```python
from build123d import *

# Parameters (mm, degrees)
F0_R     = 5.75
F1_DEPTH = 2.5
F2_R     = 1.375
F3_DEPTH = 25.4
F4_R     = 0.6
F5_DEPTH = 25.4
F6_R     = 0.6
F7_DEPTH = 25.4
F8_R     = 0.6
F9_DEPTH = 25.4
F10_SIZE = 1
F11_R    = 0.4


with BuildPart() as f1:
    # F0 (on Top) → F1 (new body)
    with BuildSketch(Plane.XY):
        with Locations((-19.332174, 0)):
            Circle(F0_R)
    extrude(amount=F1_DEPTH)

    # F2 (on face) → F3 (cut)
    with BuildSketch(Plane.XY.offset(2.5)):
        with Locations((-19.332174, 0)):
            Circle(F2_R)
    extrude(amount=-F3_DEPTH, mode=Mode.SUBTRACT)

    # F4 (on face) → F5 (cut)
    with BuildSketch(Plane.XY.offset(2.5)):
        with Locations((-22.144392, 2.014774)):
            Circle(F4_R)
    extrude(amount=-F5_DEPTH, mode=Mode.SUBTRACT)

    # F6 (on face) → F7 (cut)
    with BuildSketch(Plane.XY.offset(2.5)):
        with Locations((-19.493969, -3.397938)):
            Circle(F6_R)
    extrude(amount=-F7_DEPTH, mode=Mode.SUBTRACT)

    # F8 (on face) → F9 (cut)
    with BuildSketch(Plane.XY.offset(2.5)):
        with Locations((-16.320517, 1.792489)):
            Circle(F8_R)
    extrude(amount=-F9_DEPTH, mode=Mode.SUBTRACT)

    # F10
    f10_edges = [f1.edges().sort_by_distance(p)[0] for p in [
        (-25.082174, 0, 2.5),
    ]]
    chamfer(f10_edges, length=F10_SIZE)

    # F11
    f11_edges = [f1.edges().sort_by_distance(p)[0] for p in [
        (-25.082174, 0, 0),
    ]]
    fillet(f11_edges, radius=F11_R)


solid = f1.part
```
Verification items for the finished model (mm, model axes). Round coordinates to 2 decimals unless told otherwise and drop trailing zeros. Loops run counter-clockwise (first coordinate to the right, second up) from the corner with the lowest first, then second, coordinate; pieces in that order, holes last. Notation, with made-up numbers: (16, -36) -> (24, -36) arc R29 ccw to (24, -14) -> close; hole circle Ø11 at (53.5, 19). An arc over 180 degrees is marked (long way). Answer as a JSON object with one key per item and string values.
Q1. Section check D-D (z = 0.9). Record the boundary of the cut face in (x, y) (3 decimals), then the cut area to 3 significant figures.
Data:
{"outline": "circle Ø11.5 at (-19.332, 0); hole circle Ø1.2 at (-22.144, 2.015); hole circle Ø2.75 at (-19.332, 0); hole circle Ø1.2 at (-19.494, -3.398); hole circle Ø1.2 at (-16.321, 1.792)", "area": "94.5 mm2"}
Q2. Draft check along X on faces 1 (the cylindrical face through (-18.02, 0.41, 1.27)), 2 (the cylindrical face through (-20.093, -3.372, 1.268)), 3 (the flat face through (-18, -1, 2.5)), 4 (the cylindrical face through (-25.077, 0.253, 0.942)). Enter one of: pulls with the +X half, pulls with the -X half, needs draft (parallel to the pull), parting line crosses it, or undercut.
Data:
{"face 1": "undercut", "face 2": "undercut", "face 3": "needs draft", "face 4": "parting line crosses it"}
Q3. Scan lines: line 1 (Y direction, x = -19, z = 0.9); line 2 (Y direction, x = -19.75, z = 1.95); line 3 (X direction, y = 1.75, z = 0.9). Record each from-to range of solid material in increasing order. Write a range as from..to.
Data:
{"line 1": "y = -5.74..-3.74, -3.06..-1.33, 1.33..5.74", "line 2": "y = -5.28..-3.94, -2.86..-1.31, 1.31..5.28", "line 3": "x = -24.81..-22.68, -21.61..-16.92, -15.72..-13.85"}
Q4. Go/stop test with flat-tipped pins: P1, Ø1.1, axis at x = -19.49, y = -3.4, coming from the +Z side; P2, Ø1.5, axis at x = -21, z = 0.5, coming from the +Y side; P3, Ø1.5, axis at y = -4, z = 1.5, coming from the +X side; P4, Ø1.5, axis at y = -2.5, z = 1.5, coming from the +X side. Record where each tip stops, or that it passes through.
Data:
{"P1": "passes through", "P2": "stops at y = 5.68", "P3": "stops at x = -14.59", "P4": "stops at x = -13.85"}
Q5. Section check C-C (x = -19.5). State how many separate pieces and enclosed holes the cut face has, then the cut area to 3 significant figures.
Data:
{"separate pieces": "3", "enclosed holes": "0", "area": "17.8 mm2"}
Q6. Section check A-A (y = 0). Record the boundary of the cut face in (x, z), then the cut area to 3 significant figures.
Data:
{"outline": "(-25.08, 0.4) arc R0.4 ccw to (-24.68, 0) -> (-20.71, 0) -> (-20.71, 2.5) -> (-24.08, 2.5) -> (-25.08, 1.5) -> close; (-17.96, 0) -> (-13.98, 0) arc R0.4 ccw to (-13.58, 0.4) -> (-13.58, 1.5) -> (-14.58, 2.5) -> (-17.96, 2.5) -> close", "area": "20.8 mm2"}
Q7. Section check B-B (z = 1.85). Record the boundary of the cut face in (x, y) (3 decimals).
Data:
{"outline": "circle Ø10.8 at (-19.332, 0); hole circle Ø1.2 at (-22.144, 2.015); hole circle Ø2.75 at (-19.332, 0); hole circle Ø1.2 at (-19.494, -3.398); hole circle Ø1.2 at (-16.321, 1.792)"}
